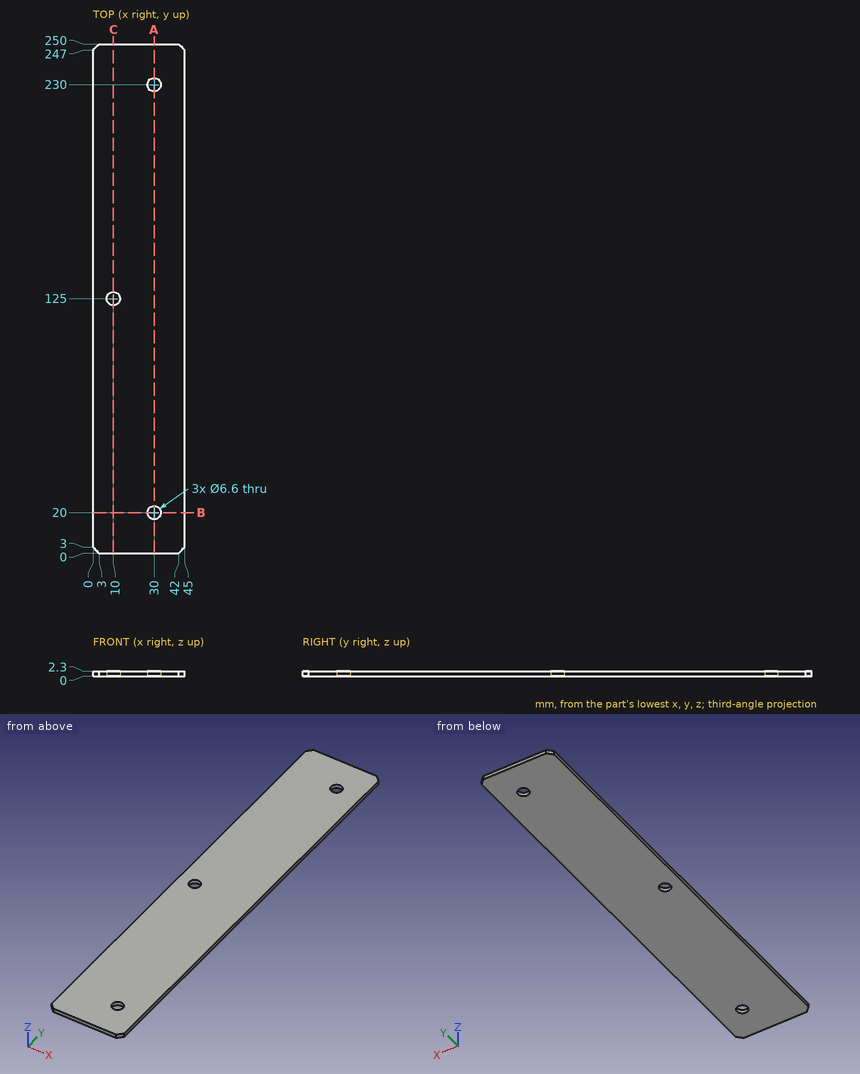
Study the drawing (mm; zero at the part's minimum x, y, z) and answer. Round coordinates to 2 decimals unless told otherwise and drop trailing zeros. Loops run counter-clockwise (first coordinate to the right, second up) from the corner with the lowest first, then second, coordinate; pieces in that order, holes last. Notation, with made-up numbers: (24.25, 52) -> (32.25, 52) arc R26 cw to (32.25, 89) -> close; hole circle Ø1 at (46.25, -34.5). An arc over 180 degrees is marked (long way). One line per item, written item: value.
1) A flat-ended cylindrical pin translates along its axis: P1, Ø5.5, axis at x = 30, y = 20, coming from the +Z side. Find the tip coordinate at first contact, or state that the pin passes through.
Answer list:
P1: passes through
2) Consider L1, parallel to Y at x = 30, z = 1.4; L2, parallel to Y at x = 10, z = 0.5; L3, parallel to X at y = 230, z = 0.8. Determine where each line is inside the solid, lowest interval first. Write a range as [from, to].
Answer list:
L1: y = [0, 16.7], [23.3, 226.7], [233.3, 250]
L2: y = [0, 121.7], [128.3, 250]
L3: x = [0, 26.7], [33.3, 45]
3) A cutting plane is placed at A-A (x = 30). Determine the outline of the cut face in (y, z), and give its area (3 significant figures).
Answer list:
outline: (0, 0) -> (16.7, 0) -> (16.7, 2.3) -> (0, 2.3) -> close; (23.3, 0) -> (226.7, 0) -> (226.7, 2.3) -> (23.3, 2.3) -> close; (233.3, 0) -> (250, 0) -> (250, 2.3) -> (233.3, 2.3) -> close
area: 545 mm²
4) A cutting plane is placed at B-B (y = 20). Determine the outline of the cut face in (x, z), and give its area (3 significant figures).
Answer list:
outline: (0, 0) -> (26.7, 0) -> (26.7, 2.3) -> (0, 2.3) -> close; (33.3, 0) -> (45, 0) -> (45, 2.3) -> (33.3, 2.3) -> close
area: 88.3 mm²
5) A cutting plane is placed at C-C (x = 10). Determine the outline of the cut face in (y, z), and give its area (3 significant figures).
Answer list:
outline: (0, 0) -> (121.7, 0) -> (121.7, 2.3) -> (0, 2.3) -> close; (128.3, 0) -> (250, 0) -> (250, 2.3) -> (128.3, 2.3) -> close
area: 560 mm²
